from build123d import *

# Parameters (mm, degrees)
SKETCH1_W                  = 760
SKETCH1_H                  = 454
BOSS_EXTRUDE1_DEPTH        = 20
SKETCH2_W                  = 740
SKETCH2_H                  = 434
CUT_EXTRUDE1_DEPTH         = 18
CONVERT_SOLID2_OUTLINE_W   = 15.7
CONVERT_SOLID2_OUTLINE_H   = 2
CONVERT_SOLID2_DEPTH       = 10.707106781
CONVERT_SOLID2_START       = 749.292893219
CONVERT_SOLID2_2_OUTLINE_W = 15.7
CONVERT_SOLID2_2_OUTLINE_H = 2
CONVERT_SOLID2_2_DEPTH     = 10.707106781
CONVERT_SOLID2_3_DEPTH     = 760
CONVERT_SOLID2_4_DEPTH     = 8
CONVERT_SOLID2_START_2     = 752
CONVERT_SOLID2_5_DEPTH     = 8
CONVERT_SOLID2_START_3     = 8
CONVERT_SOLID2_6_DEPTH     = 4.3
CONVERT_SOLID2_START_4     = 747.7
CONVERT_SOLID2_7_DEPTH     = 4.3
CONVERT_SOLID2_START_5     = 12.3
CONVERT_SOLID2_8_DEPTH     = 735.4
CONVERT_SOLID2_START_6     = -441.7
CONVERT_SOLID2_9_DEPTH     = 429.4
CONVERT_SOLID2_10_DEPTH    = 429.4


with BuildPart() as part:
    # Sketch1 → Boss-Extrude1 (new body)
    with BuildSketch(Plane(origin=(0, 0, 0), x_dir=(1, 0, 0), z_dir=(0, 1, 0))):
        with Locations((380, 227)):
            Rectangle(SKETCH1_W, SKETCH1_H)
    extrude(amount=BOSS_EXTRUDE1_DEPTH)

    # Sketch2 → Cut-Extrude1 (cut)
    with BuildSketch(Plane(origin=(0, 20, 0), x_dir=(1, 0, 0), z_dir=(0, 1, 0))):
        with Locations((380, 227)):
            Rectangle(SKETCH2_W, SKETCH2_H)
    extrude(amount=-CUT_EXTRUDE1_DEPTH, mode=Mode.SUBTRACT)

    # Convert-Solid2: read off the stored shape, not the designer's step
    # Convert-Solid2 outline → Convert-Solid2 (cut)
    with BuildSketch(Plane.YZ):
        with Locations((12.15, -9)):
            Rectangle(CONVERT_SOLID2_OUTLINE_W, CONVERT_SOLID2_OUTLINE_H)
        with Locations((12.15, -445)):
            Rectangle(CONVERT_SOLID2_OUTLINE_W, CONVERT_SOLID2_OUTLINE_H)
    extrude(amount=CONVERT_SOLID2_DEPTH, mode=Mode.SUBTRACT)

    # Convert-Solid2 2 outline → Convert-Solid2 2 (cut)
    with BuildSketch(Plane.YZ.offset(CONVERT_SOLID2_START)):
        with Locations((12.15, -9)):
            Rectangle(CONVERT_SOLID2_2_OUTLINE_W, CONVERT_SOLID2_2_OUTLINE_H)
        with Locations((12.15, -445)):
            Rectangle(CONVERT_SOLID2_2_OUTLINE_W, CONVERT_SOLID2_2_OUTLINE_H)
    extrude(amount=CONVERT_SOLID2_2_DEPTH, mode=Mode.SUBTRACT)

    # Convert-Solid2 3 outline → Convert-Solid2 3 (cut)
    with BuildSketch(Plane.YZ):
        with BuildLine():
            Line((4.3, -441.7), (2, -441.7))
            Line((2, -441.7), (2, -442.2))
            ThreePointArc((2, -442.2), (2.527207794, -443.472792206), (3.8, -444))
            Line((3.8, -444), (20, -444))
            Line((20, -444), (20, -443.292893219))
            Line((20, -443.292893219), (4.3, -443.292893219))
            Line((4.3, -443.292893219), (4.3, -441.7))
        make_face()
        with BuildLine():
            Line((2, -11.8), (2, -12.3))
            Line((2, -12.3), (4.3, -12.3))
            Line((4.3, -12.3), (4.3, -10.707106781))
            Line((4.3, -10.707106781), (20, -10.707106781))
            Line((20, -10.707106781), (20, -10))
            Line((20, -10), (3.8, -10))
            ThreePointArc((3.8, -10), (2.527207794, -10.527207794), (2, -11.8))
        make_face()
        with BuildLine():
            ThreePointArc((3.8, -446), (1.112994231, -444.887005769), (0, -442.2))
            Line((0, -442.2), (0, -454))
            Line((0, -454), (20, -454))
            Line((20, -454), (20, -446))
            Line((20, -446), (3.8, -446))
        make_face()
        with BuildLine():
            Line((0, 0), (0, -11.8))
            ThreePointArc((0, -11.8), (1.112994231, -9.112994231), (3.8, -8))
            Line((3.8, -8), (20, -8))
            Line((20, -8), (20, 0))
            Line((20, 0), (0, 0))
        make_face()
    extrude(amount=CONVERT_SOLID2_3_DEPTH, mode=Mode.SUBTRACT)

    # Convert-Solid2 4 outline → Convert-Solid2 4 (cut)
    with BuildSketch(Plane.YZ):
        with BuildLine():
            Line((2, -442.2), (2, -441.7))
            Line((2, -441.7), (4.3, -441.7))
            Line((4.3, -441.7), (4.3, -443.292893219))
            Line((4.3, -443.292893219), (20, -443.292893219))
            Line((20, -443.292893219), (20, -10.707106781))
            Line((20, -10.707106781), (4.3, -10.707106781))
            Line((4.3, -10.707106781), (4.3, -12.3))
            Line((4.3, -12.3), (2, -12.3))
            Line((2, -12.3), (2, -11.8))
            ThreePointArc((2, -11.8), (2.527207794, -10.527207794), (3.8, -10))
            Line((3.8, -10), (4.3, -10))
            Line((4.3, -10), (4.3, -8))
            Line((4.3, -8), (3.8, -8))
            ThreePointArc((3.8, -8), (1.112994231, -9.112994231), (0, -11.8))
            Line((0, -11.8), (0, -442.2))
            ThreePointArc((0, -442.2), (1.112994231, -444.887005769), (3.8, -446))
            Line((3.8, -446), (4.3, -446))
            Line((4.3, -446), (4.3, -444))
            Line((4.3, -444), (3.8, -444))
            ThreePointArc((3.8, -444), (2.527207794, -443.472792206), (2, -442.2))
        make_face()
    extrude(amount=CONVERT_SOLID2_4_DEPTH, mode=Mode.SUBTRACT)

    # Convert-Solid2 5 outline → Convert-Solid2 5 (cut)
    with BuildSketch(Plane.YZ.offset(CONVERT_SOLID2_START_2)):
        with BuildLine():
            Line((2, -442.2), (2, -441.7))
            Line((2, -441.7), (4.3, -441.7))
            Line((4.3, -441.7), (4.3, -443.292893219))
            Line((4.3, -443.292893219), (20, -443.292893219))
            Line((20, -443.292893219), (20, -10.707106781))
            Line((20, -10.707106781), (4.3, -10.707106781))
            Line((4.3, -10.707106781), (4.3, -12.3))
            Line((4.3, -12.3), (2, -12.3))
            Line((2, -12.3), (2, -11.8))
            ThreePointArc((2, -11.8), (2.527207794, -10.527207794), (3.8, -10))
            Line((3.8, -10), (4.3, -10))
            Line((4.3, -10), (4.3, -8))
            Line((4.3, -8), (3.8, -8))
            ThreePointArc((3.8, -8), (1.112994231, -9.112994231), (0, -11.8))
            Line((0, -11.8), (0, -442.2))
            ThreePointArc((0, -442.2), (1.112994231, -444.887005769), (3.8, -446))
            Line((3.8, -446), (4.3, -446))
            Line((4.3, -446), (4.3, -444))
            Line((4.3, -444), (3.8, -444))
            ThreePointArc((3.8, -444), (2.527207794, -443.472792206), (2, -442.2))
        make_face()
    extrude(amount=CONVERT_SOLID2_5_DEPTH, mode=Mode.SUBTRACT)

    # Convert-Solid2 6 outline → Convert-Solid2 6 (cut)
    with BuildSketch(Plane.YZ.offset(CONVERT_SOLID2_START_3)):
        with BuildLine():
            Line((2, -442.2), (2, -441.7))
            Line((2, -441.7), (0, -441.7))
            Line((0, -441.7), (0, -442.2))
            ThreePointArc((0, -442.2), (1.112994231, -444.887005769), (3.8, -446))
            Line((3.8, -446), (4.3, -446))
            Line((4.3, -446), (4.3, -444))
            Line((4.3, -444), (3.8, -444))
            ThreePointArc((3.8, -444), (2.527207794, -443.472792206), (2, -442.2))
        make_face()
        with BuildLine():
            Line((0, -12.3), (2, -12.3))
            Line((2, -12.3), (2, -11.8))
            ThreePointArc((2, -11.8), (2.527207794, -10.527207794), (3.8, -10))
            Line((3.8, -10), (4.3, -10))
            Line((4.3, -10), (4.3, -8))
            Line((4.3, -8), (3.8, -8))
            ThreePointArc((3.8, -8), (1.112994231, -9.112994231), (0, -11.8))
            Line((0, -11.8), (0, -12.3))
        make_face()
    extrude(amount=CONVERT_SOLID2_6_DEPTH, mode=Mode.SUBTRACT)

    # Convert-Solid2 7 outline → Convert-Solid2 7 (cut)
    with BuildSketch(Plane.YZ.offset(CONVERT_SOLID2_START_4)):
        with BuildLine():
            Line((2, -442.2), (2, -441.7))
            Line((2, -441.7), (0, -441.7))
            Line((0, -441.7), (0, -442.2))
            ThreePointArc((0, -442.2), (1.112994231, -444.887005769), (3.8, -446))
            Line((3.8, -446), (4.3, -446))
            Line((4.3, -446), (4.3, -444))
            Line((4.3, -444), (3.8, -444))
            ThreePointArc((3.8, -444), (2.527207794, -443.472792206), (2, -442.2))
        make_face()
        with BuildLine():
            Line((0, -12.3), (2, -12.3))
            Line((2, -12.3), (2, -11.8))
            ThreePointArc((2, -11.8), (2.527207794, -10.527207794), (3.8, -10))
            Line((3.8, -10), (4.3, -10))
            Line((4.3, -10), (4.3, -8))
            Line((4.3, -8), (3.8, -8))
            ThreePointArc((3.8, -8), (1.112994231, -9.112994231), (0, -11.8))
            Line((0, -11.8), (0, -12.3))
        make_face()
    extrude(amount=CONVERT_SOLID2_7_DEPTH, mode=Mode.SUBTRACT)

    # Convert-Solid2 8 outline → Convert-Solid2 8 (add)
    with BuildSketch(Plane.YZ.offset(CONVERT_SOLID2_START_5)):
        with BuildLine():
            ThreePointArc((3.8, -444), (2.527207794, -443.472792206), (2, -442.2))
            Line((2, -442.2), (2, -444))
            Line((2, -444), (3.8, -444))
        make_face()
        with BuildLine():
            Line((2, -10), (2, -11.8))
            ThreePointArc((2, -11.8), (2.527207794, -10.527207794), (3.8, -10))
            Line((3.8, -10), (2, -10))
        make_face()
    extrude(amount=CONVERT_SOLID2_8_DEPTH)

    # Convert-Solid2 9 outline → Convert-Solid2 9 (cut)
    with BuildSketch(Plane.XY.offset(CONVERT_SOLID2_START_6)):
        with BuildLine():
            Line((752, 0), (752, 3.8))
            ThreePointArc((752, 3.8), (750.887005769, 1.112994231), (748.2, 0))
            Line((748.2, 0), (752, 0))
        make_face()
        with BuildLine():
            Line((8, 0), (11.8, 0))
            ThreePointArc((11.8, 0), (9.112994231, 1.112994231), (8, 3.8))
            Line((8, 3.8), (8, 0))
        make_face()
    extrude(amount=CONVERT_SOLID2_9_DEPTH, mode=Mode.SUBTRACT)

    # Convert-Solid2 10 outline → Convert-Solid2 10 (add)
    with BuildSketch(Plane.XY.offset(CONVERT_SOLID2_START_6)):
        with BuildLine():
            Line((750, 2), (750, 3.8))
            ThreePointArc((750, 3.8), (749.472792206, 2.527207794), (748.2, 2))
            Line((748.2, 2), (750, 2))
        make_face()
        with BuildLine():
            Line((10, 2), (11.8, 2))
            ThreePointArc((11.8, 2), (10.527207794, 2.527207794), (10, 3.8))
            Line((10, 3.8), (10, 2))
        make_face()
    extrude(amount=CONVERT_SOLID2_10_DEPTH)


solid = part.part
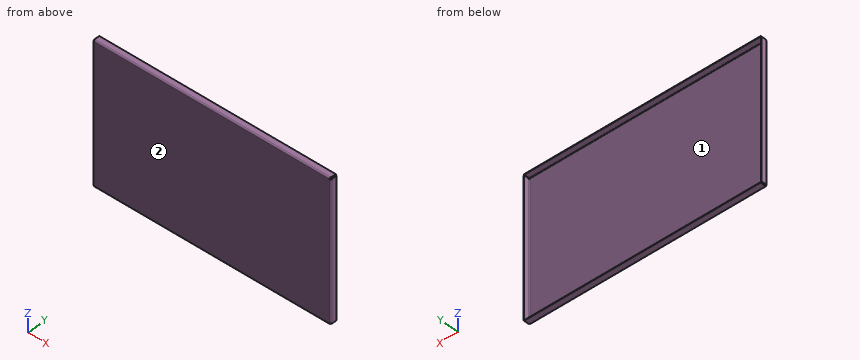
For this review, take the finished solid that the model builds, in its own axes (mm). Face numbers are marked on the shaded views. Give positions to 0.01 mm unless a question says otherwise; leave off trailing zeros. Order: outer loops, then holes, each group sorted by start corner. A loop starts at its lowest first (then second) coordinate and runs counter-clockwise, first axis right, second up. Notation, with made-up numbers: (0, -20) - (36, -20) arc R5 ccw to (36, -12) - close; hole circle Ø5 at (-19.5, 42). An arc over 180 degrees is marked (long way). Answer as a JSON object with one key per item and string values. Group by question number.
Item 1: Take a section at C-C on z = -86. Give the boundary of the cut face in (x, y), and give its area (3 significant figures).
Item 2: Draft analysis for pull direction X (two halves, no side actions). For the marked faces 1 and 2, state which applies: pulls with the +X half, pulls with the -X half, needs draft (parallel to the pull), parting line crosses it, or undercut.
Item 3: Take a section at A-A on y = 8.75. Give the boundary of the cut face in (x, z), and give its area (3 significant figures).
Item 4: Take a section at B-B on x = 304. Give the boundary of the cut face in (y, z), and give its area (3 significant figures).
Item 5: Wall thickness on line 1 along X through (y, z) = (17.75, -45.5); line 2 along Z through (x, y) = (465.5, 13); line 3 along Y through (x, z) = (719, -291.5): over which ranges is each line inside the solid? List them lowest first.
Item 6: Clearance check with flat-ended pins moving along their axes: pin 1 Ø6 at (x, z) = (261.5, -402) entering from +Y; pin 2 Ø1.6 at (x, y) = (9, 16) entering from +Z; pin 3 Ø2 at (y, z) = (3, -10) entering from +X; pin 4 Ø4.5 at (x, y) = (749, 3) entering from -Z. State where each tip first meets the part, or that it passes through.
Reported:
{
 "1": {"outline": "(8, 3.8) arc R3.8 ccw to (11.8, 0) - (748.2, 0) arc R3.8 ccw to (752, 3.8) - (752, 20) - (750, 20) - (750, 3.8) arc R1.8 cw to (748.2, 2) - (11.8, 2) arc R1.8 cw to (10, 3.8) - (10, 20) - (8, 20) - close", "area": "1,560 mm^2"},
 "2": {"face 1": "undercut", "face 2": "needs draft"},
 "3": {"outline": "(8, -443.29) - (10, -443.29) - (10, -10.71) - (8, -10.71) - close; (10.71, -446) - (749.29, -446) - (749.29, -444) - (10.71, -444) - close; (10.71, -10) - (749.29, -10) - (749.29, -8) - (10.71, -8) - close; (750, -443.29) - (752, -443.29) - (752, -10.71) - (750, -10.71) - close", "area": "4,680 mm^2"},
 "4": {"outline": "(0, -442.2) arc R3.8 ccw to (3.8, -446) - (20, -446) - (20, -444) - (3.8, -444) arc R1.8 cw to (2, -442.2) - (2, -11.8) arc R1.8 cw to (3.8, -10) - (20, -10) - (20, -8) - (3.8, -8) arc R3.8 ccw to (0, -11.8) - close", "area": "943 mm^2"},
 "5": {"line 1": "8 to 10, 750 to 752", "line 2": "-446 to -444, -10 to -8", "line 3": "0 to 2"},
 "6": {"pin 1": "y = 2", "pin 2": "z = -10.71", "pin 3": "x = 747.7", "pin 4": "z = -446"}
}
